from build123d import *

# Parameters (mm, degrees)
F0_R      = 12.7
F1_DEPTH  = 30.1625
F4_R      = 5.08
F5_R      = 7.62
F6_R      = 5.08
F7_DEPTH  = 41.275
F9_DEPTH  = 19.05
F10_R     = 5.08
F11_W     = 22.352
F11_H     = 22.3266
F11_W_2   = 21.9653917967
F11_W_3   = 4.9921344993
F12_DEPTH = 57.151
F13_R     = 6.35
F14_DEPTH = 22.353


# Not quite as in the source:
# - a feature names something its author has since deleted; it is built from what else it names


with BuildPart() as f1:
    # F0 (on Front) → F1 (new body, symmetric)
    with BuildSketch(Plane.XZ):
        with BuildLine():
            Line((11.6077999467, 0), (5.6133999467, 22.352))
            Line((5.6133999467, 22.352), (-57.8866000533, 22.352))
            ThreePointArc((-57.8866000533, 22.352), (-64.4333492802, 6.5467492269), (-80.2386000533, 0))
            Line((-80.2386000533, 0), (11.6077999467, 0))
        make_face()
        Polygon((69.6339349389, 22.352), (37.0077999467, 22.352), (37.0077999467, 0), (69.4951486566, 0), align=None)
        Polygon((113.9697999467, 22.352), (69.6339349389, 22.352), (69.4951486566, 0), (113.9697999467, 0), align=None)
        with BuildLine():
            ThreePointArc((-80.2386000533, 0), (-64.4333492802, 6.5467492269), (-57.8866000533, 22.352))
            ThreePointArc((-57.8866000533, 22.352), (-96.0438508264, 38.1572507731), (-80.2386000533, 0))
        make_face()
        with Locations((-80.2386000533, 22.352)):
            Circle(F0_R, mode=Mode.SUBTRACT)
        Polygon((37.0077999467, 0), (37.0077999467, 22.352), (5.6133999467, 22.352), (11.6077999467, 0), align=None)
        with BuildLine():
            ThreePointArc((50.7999999467, 57.15), (47.2258153083, 38.4343576341), (37.0077999467, 22.352))
            Line((37.0077999467, 22.352), (69.6339349389, 22.352))
            Line((69.6339349389, 22.352), (69.8499999467, 57.15))
            Line((69.8499999467, 57.15), (50.7999999467, 57.15))
        make_face()
    extrude(amount=F1_DEPTH, both=True)

    # F4
    f4_edges = [f1.edges().sort_by_distance(p)[0] for p in [
        (69.85, 0, 57.15),
    ]]
    fillet(f4_edges, radius=F4_R)

    # F5
    f5_edges = [f1.edges().sort_by_distance(p)[0] for p in [
        (113.9698, 0, 22.352),
    ]]
    fillet(f5_edges, radius=F5_R)

    # F6
    f6_edges = [f1.edges().sort_by_distance(p)[0] for p in [
        (-57.8866, 0, 22.352),
    ]]
    fillet(f6_edges, radius=F6_R)

    # F3 (on face) → F7 (cut)
    with BuildSketch(Plane(origin=(0, 30.1625, 0), x_dir=(-1, 0, 0), z_dir=(0, 1, 0))):
        with BuildLine():
            Line((-69.8499999467, 57.15), (-69.6339349389, 22.352))
            Line((-69.6339349389, 22.352), (-37.0077999467, 22.352))
            ThreePointArc((-37.0077999467, 22.352), (-47.2258153083, 38.4343576341), (-50.7999999467, 57.15))
            Line((-50.7999999467, 57.15), (-69.8499999467, 57.15))
        make_face()
    extrude(amount=-F7_DEPTH, mode=Mode.SUBTRACT)

    # F2 (on face) → F9 (cut)
    with BuildSketch(Plane.XZ.offset(30.1625)):
        Polygon((37.0077999467, 22.352), (5.6133999467, 22.352), (11.6077999467, 0), (37.0077999467, 0), align=None)
    extrude(amount=-F9_DEPTH, mode=Mode.SUBTRACT)

    # F10
    f10_edges = [f1.edges().sort_by_distance(p)[0] for p in [
        (69.633935, -20.6375, 22.352),
    ]]
    fillet(f10_edges, radius=F10_R)

    # F11 (on Top) → F12 (cut, through all)
    with BuildSketch(Plane.XY):
        with Locations((-91.4146000533, 0)):
            Rectangle(F11_W, F11_H)
        with Locations((-69.2559041549, 0)):
            Rectangle(F11_W_2, F11_H)
        with Locations((-55.7771410069, 0)):
            Rectangle(F11_W_3, F11_H)
    extrude(amount=F12_DEPTH, mode=Mode.SUBTRACT)

    # F13 (on face) → F14 (cut, through all)
    with BuildSketch(Plane.XY.offset(22.352)):
        with Locations((75.1077999467, 7.8105)):
            Circle(F13_R)
    extrude(amount=-F14_DEPTH, mode=Mode.SUBTRACT)


solid = f1.part
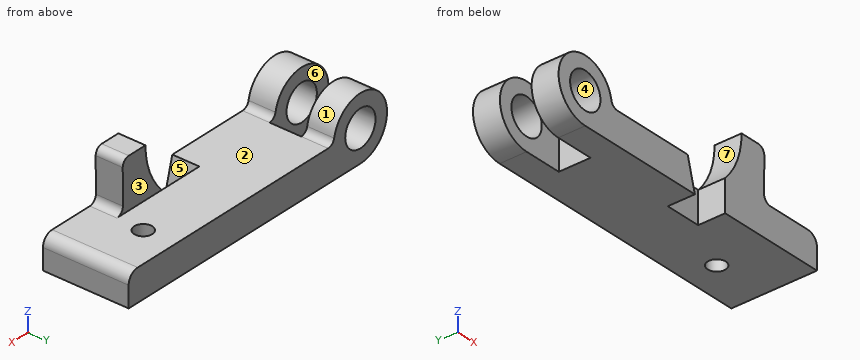
Geometry: final body of the model. Coordinates: model frame, mm. Face numbers are marked on the shaded views. A direction names the side the tool comes from. Round coordinates to 2 decimals unless told otherwise and drop trailing zeros. Loops run counter-clockwise (first coordinate to the right, second up) from the corner with the lowest first, then second, coordinate; pieces in that order, holes last. Notation, with made-up numbers: M 53,-37.75 L 78,-37.75 A21 cw 78,-10.75 Z; hole C 31.5,50 d8. An arc over 180 degrees is marked long. Put each result on its own line as item: value. Start each with the question number.
(1) Contact query for flat-ended pins moving along their axis: pin 1 Ø8 at (x, y) = (17, -10.5) entering from +Z; pin 2 Ø12 at (y, z) = (-12.5, 41.5) entering from -X; pin 3 Ø11 at (y, z) = (-1, 8.5) entering from -X. Output: stop coordinate, or through.
(2) Set-up query: the marked faces 5, 6 and 7. Return all of +Z, -Z, +X, -X, +Y, -Y with unobstructed straight access to the full face (end or side cutting, diameter ignored); none if empty.
(3) Section query C-C (y = 20). Return loops of the section in (x, z).
(4) Material intervals for line 1 along X through (y, z) = (-13, 26); line 2 along X through (y, z) = (-28, 20.5); line 3 along Z through (x, y) = (-2, -24), sorted ascending. Write a range as [from, to].
(5) Draft query along Z for the marked faces 1, 2, 3 and 4. Return one class per face: +Z half, -Z half, draft (parallel to the pull), parting line (faces both ways), or undercut.
(6) Section query B-B (z = 17.5). Return loops of the section in (x, y).
(7) Section query D-D (z = 4.5). Return loops of the section in (x, y), then the cut area to 3 significant figures.
(8) Section query A-A (y = -16). Return loops of the section in (x, z), then the cut area to 3 significant figures.
Findings below:
1. pin 1: stops at z = 22.35
1. pin 2: stops at x = -98.31
1. pin 3: stops at x = -53.28
2. face 5: +Z, -Y
2. face 6: +Z, -Z, -X
2. face 7: +Z, +Y, -Y
3. outline: M -80.24,0 L 113.97,0 L 113.97,14.73 A7.62 ccw 106.35,22.35 L -53.28,22.35 A5.08 cw -58.27,26.49 A22.35 ccw long Z; hole C -80.24,22.35 d25.4
4. line 1: x = [-102.29, -92.4], [-68.07, -58.16], [40.13, 69.87]
4. line 2: x = [-102.51, -92.8], [-67.67, 6.11], [37.01, 111.33]
4. line 3: z = [0, 22.35]
5. face 1: parting line
5. face 2: +Z half
5. face 3: draft
5. face 4: undercut
6. outline: M -102.06,-30.16 L -91.98,-30.16 L -91.98,-11.16 L -102.06,-11.16 Z; M -102.06,11.16 L -91.98,11.16 L -91.98,30.16 L -102.06,30.16 Z; M -68.5,-30.16 L 6.91,-30.16 L 6.91,-11.11 L 37.01,-11.11 L 37.01,-30.16 L 113.45,-30.16 L 113.45,30.16 L -68.5,30.16 L -68.5,11.16 L -53.28,11.16 L -53.28,-11.16 L -68.5,-11.16 Z; hole C 75.11,7.81 d12.7
7. outline: M -93.69,-30.16 L 10.4,-30.16 L 10.4,-11.11 L 37.01,-11.11 L 37.01,-30.16 L 113.97,-30.16 L 113.97,30.16 L -93.69,30.16 L -93.69,11.16 L -53.28,11.16 L -53.28,-11.16 L -93.69,-11.16 Z; hole C 75.11,7.81 d12.7
7. area: 11,000 mm2
8. outline: M -80.24,0 L 11.61,0 L 5.61,22.35 L -53.28,22.35 A5.08 cw -58.27,26.49 A22.35 ccw long Z; M 37.01,0 L 113.97,0 L 113.97,14.73 A7.62 ccw 106.35,22.35 L 74.75,22.35 A5.08 cw 69.67,27.46 L 69.82,52.04 A5.08 ccw 64.74,57.15 L 50.8,57.15 A50.8 cw 37.01,22.35 Z; hole C -80.24,22.35 d25.4
8. area: 5,180 mm2
